Geometry check sheet. Reference: the model listing, model coordinates, mm. Face numbers are marked on the shaded views. A direction names the side the tool comes from. Give positions to 0.01 mm unless a question says otherwise; leave off trailing zeros. Loops run counter-clockwise (first coordinate to the right, second up) from the corner with the lowest first, then second, coordinate; pieces in that order, holes last. Notation, with made-up numbers: (72, 62.5) -> (125, 62.5) arc R7 cw to (125, 70.5) -> close; hole circle Ø4 at (66, 56). An arc over 180 degrees is marked (long way). One line per item, written item: value. Start each with the question number.
(1) Sectioned sample at C-C, the plane x = -34. Record the cut outline in (y, z), then the cut area to 3 significant figures.
(2) Tool access check on the marked faces 3 and 4. Record the directions out of +Z, -Z, +X, -X, +Y, -Y that give a thin tool (end or side, any length) a straight path to the whole face; none if there is none.
(3) Gauge pin test, flat ends, axial feed: pin 1 Ø0.8 at (x, z) = (-15, 0.5) entering from +Y; pin 2 Ø1.1 at (x, z) = (-9.5, 1) entering from +Y; pin 3 Ø10 at (x, y) = (-27, 14) entering from +Z. Record the tip position at first contact, or that the pin passes through.
(4) Scan lines: line 1 along Y through (x, z) = (0, -0.05); line 2 along Y through (x, z) = (0, -1); line 3 along Y through (x, z) = (-4.5, 1.2). Record each from-to range of solid material in increasing order. Write a range as from..to.
(5) Sectioned sample at A-A, the plane y = 0. Record the cut outline in (x, z).
(6) Draft check along Y on the marked faces 1 and 2. Enter one of: pulls with the +Y half, pulls with the -Y half, needs draft (parallel to the pull), parting line crosses it, or undercut.
(7) Sectioned sample at D-D, the plane y = -12.5. Record the cut outline in (x, z).
(8) Sectioned sample at B-B, the plane x = -1.5. Record the cut outline in (y, z).
from build123d import *

# Parameters (mm, degrees)
CYLINDER_R        = 1.1
CYLINDER_DEPTH    = 27
ARRAY018_Y_COUNT  = 2
ARRAY018_Y_PITCH  = 64.8
BOX_W             = 5
BOX_H             = 2.6
BOX_DEPTH         = 10
ARRAY019_X_COUNT  = 3
ARRAY019_X_PITCH  = 11
ARRAY019_Y_COUNT  = 2
ARRAY019_Y_PITCH  = 64.8
ARRAY017_X_COUNT  = 2
ARRAY017_X_PITCH  = 3
ARRAY017_Y_COUNT  = 2
ARRAY017_Y_PITCH  = 64.8
BOX030_W          = 1.8
BOX030_H          = 68
BOX030_DEPTH      = 10
BOX029_W          = 37
BOX029_H          = 1.8
BOX029_DEPTH      = 10
ARRAY016_Y_COUNT  = 2
ARRAY016_Y_PITCH  = 66.2
CYLINDER021_R     = 6
CYLINDER021_DEPTH = 10
CYLINDER022_R     = 7
CYLINDER022_DEPTH = 10
CYLINDER020_R     = 6
CYLINDER020_DEPTH = 10
BOX028_W          = 22
BOX028_H          = 58
BOX028_DEPTH      = 1.5
BOX027_W          = 52
BOX027_H          = 29
BOX027_DEPTH      = 1.5
BOX026_W          = 52
BOX026_H          = 62
BOX026_DEPTH      = 1
FILLET018_R       = 2.5
FILLET019_R       = 10.5
CYLINDER019_W     = 15.5
CYLINDER019_H     = 3.1
CYLINDER019_ANGLE = 90
BOX024_W          = 15.5
BOX024_H          = 37
BOX024_DEPTH      = 3.1
BOX025_W          = 43.5
BOX025_H          = 68
BOX025_DEPTH      = 3.1
FILLET017_R       = 2
CYLINDER018_W     = 15.5
CYLINDER018_H     = 3.1
CYLINDER018_ANGLE = 90
FILLET020_R       = 1


with BuildPart() as array018:
    # Cylinder → Cylinder (new body)
    with BuildSketch(Plane(origin=(-40.5, -32.4, 0.2), x_dir=(0, 0, -1), z_dir=(1, 0, 0))):
        Circle(CYLINDER_R)
    extrude(amount=CYLINDER_DEPTH)

    # Array018 Y: Array018 ×2


with BuildPart() as array018_1:
    add(array018.part)
    with Locations(*[(0, i * ARRAY018_Y_PITCH, 0) for i in range(1, ARRAY018_Y_COUNT)]):
        add(array018.part)


with BuildPart() as array019:
    # Box → Box (new body)
    with BuildSketch(Plane(origin=(-18.5, -33.5, 0.2), x_dir=(1, 0, 0), z_dir=(0, 0, 1))):
        with Locations((2.5, 1.3)):
            Rectangle(BOX_W, BOX_H)
    extrude(amount=BOX_DEPTH)

    # Array019 X: Array019 ×3


with BuildPart() as array019_1:
    add(array019.part)
    with Locations(*[(-i * ARRAY019_X_PITCH, 0, 0) for i in range(1, ARRAY019_X_COUNT)]):
        add(array019.part)

    # Array019 Y: Array019 ×2


with BuildPart() as array019_2:
    add(array019_1.part)
    with Locations(*[(0, i * ARRAY019_Y_PITCH, 0) for i in range(1, ARRAY019_Y_COUNT)]):
        add(array019_1.part)


with BuildPart() as obj1:
    # Sphere001 → Sphere001 (revolve)
    with BuildSketch(Plane(origin=(-10.5, -32.4, 0.2), x_dir=(1, 0, 0), z_dir=(0, -1, 0))):
        with BuildLine():
            ThreePointArc((0, -1.1), (1.1, 0), (0, 1.1))
            Line((0, 1.1), (0, -1.1))
        make_face()
    revolve(axis=Axis((-10.5, -32.4, 0.2), (0, 0, 1)))

    # Array017 X: obj1_2


with BuildPart() as obj1_1:
    add(obj1.part)
    with Locations(*[(-i * ARRAY017_X_PITCH, 0, 0) for i in range(1, ARRAY017_X_COUNT)]):
        add(obj1.part)

    # Array017 Y: obj1_2


with BuildPart() as obj1_2:
    add(obj1_1.part)
    with Locations(*[(0, i * ARRAY017_Y_PITCH, 0) for i in range(1, ARRAY017_Y_COUNT)]):
        add(obj1_1.part)

    # Fusion013: union Array018, Array019
    add(array018_1.part)
    add(array019_2.part)


with BuildPart() as obj2:
    # Box030 → Box030 (new body)
    with BuildSketch(Plane(origin=(-43.5, -34, -1.4), x_dir=(1, 0, 0), z_dir=(0, 0, 1))):
        with Locations((0.9, 34)):
            Rectangle(BOX030_W, BOX030_H)
    extrude(amount=BOX030_DEPTH)


with BuildPart() as obj3:
    # Box029 → Box029 (new body)
    with BuildSketch(Plane(origin=(-43.5, -34, -1.4), x_dir=(1, 0, 0), z_dir=(0, 0, 1))):
        with Locations((18.5, 0.9)):
            Rectangle(BOX029_W, BOX029_H)
    extrude(amount=BOX029_DEPTH)

    # Array016 Y: obj3 ×2


with BuildPart() as obj3_1:
    add(obj3.part)
    with Locations(*[(0, i * ARRAY016_Y_PITCH, 0) for i in range(1, ARRAY016_Y_COUNT)]):
        add(obj3.part)

    # Fusion012: union obj2
    add(obj2.part)


with BuildPart() as obj4:
    # Cylinder021 → Cylinder021 (new body)
    with BuildSketch(Plane(origin=(0, 21.5, -3), x_dir=(1, 0, 0), z_dir=(0, 0, 1))):
        Circle(CYLINDER021_R)
    extrude(amount=CYLINDER021_DEPTH)


with BuildPart() as obj5:
    # Cylinder022 → Cylinder022 (new body)
    with BuildSketch(Plane.XY.offset(-3)):
        Circle(CYLINDER022_R)
    extrude(amount=CYLINDER022_DEPTH)


with BuildPart() as obj6:
    # Cylinder020 → Cylinder020 (new body)
    with BuildSketch(Plane(origin=(0, -21.5, -3), x_dir=(1, 0, 0), z_dir=(0, 0, 1))):
        Circle(CYLINDER020_R)
    extrude(amount=CYLINDER020_DEPTH)

    # Fusion009: union obj4, obj5
    add(obj4.part)
    add(obj5.part)


with BuildPart() as partcut2:
    # Box028 → Box028 (new body)
    with BuildSketch(Plane(origin=(-39, -29, -0.8), x_dir=(1, 0, 0), z_dir=(0, 0, 1))):
        with Locations((11, 29)):
            Rectangle(BOX028_W, BOX028_H)
    extrude(amount=BOX028_DEPTH)


with BuildPart() as partcuts:
    # Box027 → Box027 (new body)
    with BuildSketch(Plane(origin=(-41, -14.5, -0.8), x_dir=(1, 0, 0), z_dir=(0, 0, 1))):
        with Locations((26, 14.5)):
            Rectangle(BOX027_W, BOX027_H)
    extrude(amount=BOX027_DEPTH)

    # Fusion008: union PartCut2
    add(partcut2.part)


with BuildPart() as fillet019:
    # Box026 → Box026 (new body)
    with BuildSketch(Plane(origin=(-41, -31, 0.7), x_dir=(1, 0, 0), z_dir=(0, 0, 1))):
        with Locations((26, 31)):
            Rectangle(BOX026_W, BOX026_H)
    extrude(amount=BOX026_DEPTH)

    # Fillet018
    fillet018_edges = [fillet019.edges().sort_by_distance(p)[0] for p in [
        (-41, -31, 1.2),
        (-41, 31, 1.2),
    ]]
    fillet(fillet018_edges, radius=FILLET018_R)

    # Fillet019
    fillet019_edges = [fillet019.edges().sort_by_distance(p)[0] for p in [
        (11, -31, 1.2),
        (11, 31, 1.2),
    ]]
    fillet(fillet019_edges, radius=FILLET019_R)


with BuildPart() as obj7:
    # Cylinder019 → Cylinder019 (revolve)
    with BuildSketch(Plane(origin=(0, -18.5, -1.4), x_dir=(0, -1, 0), z_dir=(-1, 0, 0))):
        with Locations((7.75, 1.55)):
            Rectangle(CYLINDER019_W, CYLINDER019_H)
    revolve(axis=Axis((0, -18.5, -1.4), (0, 0, 1)), revolution_arc=CYLINDER019_ANGLE)


with BuildPart() as obj8:
    # Box024 → Box024 (new body)
    with BuildSketch(Plane(origin=(0, -18.5, -1.4), x_dir=(1, 0, 0), z_dir=(0, 0, 1))):
        with Locations((7.75, 18.5)):
            Rectangle(BOX024_W, BOX024_H)
    extrude(amount=BOX024_DEPTH)


with BuildPart() as fillet017:
    # Box025 → Box025 (new body)
    with BuildSketch(Plane(origin=(-43.5, -34, -1.4), x_dir=(1, 0, 0), z_dir=(0, 0, 1))):
        with Locations((21.75, 34)):
            Rectangle(BOX025_W, BOX025_H)
    extrude(amount=BOX025_DEPTH)

    # Fillet017
    fillet017_edges = [fillet017.edges().sort_by_distance(p)[0] for p in [
        (-43.5, -34, 0.15),
        (-43.5, 34, 0.15),
    ]]
    fillet(fillet017_edges, radius=FILLET017_R)


with BuildPart() as obj9:
    # Cylinder018 → Cylinder018 (revolve)
    with BuildSketch(Plane(origin=(0, 18.5, -1.4), x_dir=(1, 0, 0), z_dir=(0, -1, 0))):
        with Locations((7.75, 1.55)):
            Rectangle(CYLINDER018_W, CYLINDER018_H)
    revolve(axis=Axis((0, 18.5, -1.4), (0, 0, 1)), revolution_arc=CYLINDER018_ANGLE)

    # Fusion007: union obj7, obj8, Fillet017
    add(obj7.part)
    add(obj8.part)
    add(fillet017.part)

    # Cut030: cut Fillet019
    add(fillet019.part, mode=Mode.SUBTRACT)

    # Cut031: cut PartCuts
    add(partcuts.part, mode=Mode.SUBTRACT)

    # Cut032: cut obj6
    add(obj6.part, mode=Mode.SUBTRACT)

    # Cut033: cut obj3
    add(obj3_1.part, mode=Mode.SUBTRACT)

    # Fillet020
    fillet020_edges = [obj9.edges().sort_by_distance(p)[0] for p in [
        (-6.5, 34, 0.15),
        (-6.5, -34, 0.15),
        (-41.7, -32.2, 0.15),
        (-41.7, 32.2, 0.15),
    ]]
    fillet(fillet020_edges, radius=FILLET020_R)

    # Cut: cut obj1
    add(obj1_2.part, mode=Mode.SUBTRACT)


solid = obj9.part
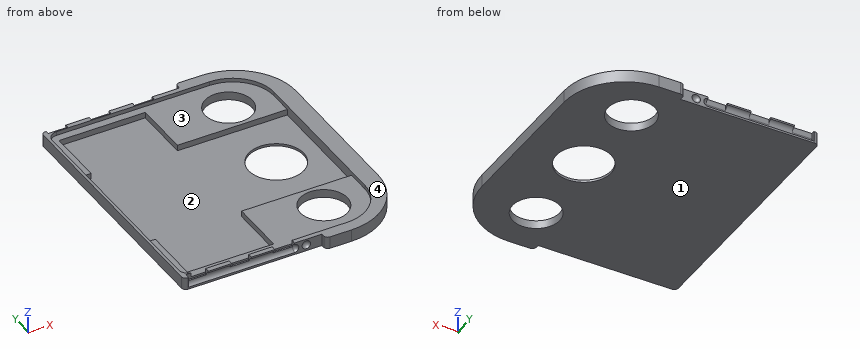
Calculated:
1. outline: (-32.2, -1.4) -> (32.2, -1.4) -> (32.2, -0.88) arc R1.1 cw to (32.2, 1.28) -> (32.2, 1.7) -> (31, 1.7) -> (31, 0.7) -> (29, 0.7) -> (29, -0.8) -> (-29, -0.8) -> (-29, 0.7) -> (-31, 0.7) -> (-31, 1.7) -> (-32.2, 1.7) -> (-32.2, 1.28) arc R1.1 cw to (-32.2, -0.88) -> close
1. area: 47.7 mm2
2. face 3: +Z
2. face 4: +Z, +X, -X, +Y, -Y
3. pin 1: stops at y = 31.3
3. pin 2: stops at y = 32.2
3. pin 3: stops at z = -0.8
4. line 1: y = -34..-27.5, -15.5..-14.5, 14.5..15.5, 27.5..34
4. line 2: y = -34..-27.5, -15.5..-7, 7..15.5, 27.5..34
4. line 3: y = -34..-31, 31..34
5. outline: (-41.7, -1.4) -> (-7, -1.4) -> (-7, -0.8) -> (-41, -0.8) -> (-41, 1.7) -> (-41.7, 1.7) -> close; (7, -1.4) -> (15.5, -1.4) -> (15.5, 1.7) -> (11, 1.7) -> (11, -0.8) -> (7, -0.8) -> close
6. face 1: needs draft
6. face 2: undercut
7. outline: (-41.7, -1.4) -> (15.5, -1.4) -> (15.5, 1.7) -> (11, 1.7) -> (11, -0.8) -> (-41, -0.8) -> (-41, 1.7) -> (-41.7, 1.7) -> close
8. outline: (-34, -1.4) -> (-27.31, -1.4) -> (-27.31, 0.7) -> (-31, 0.7) -> (-31, 1.7) -> (-34, 1.7) -> close; (-15.69, -1.4) -> (-6.84, -1.4) -> (-6.84, -0.8) -> (-14.5, -0.8) -> (-14.5, 0.7) -> (-15.69, 0.7) -> close; (6.84, -1.4) -> (15.69, -1.4) -> (15.69, 0.7) -> (14.5, 0.7) -> (14.5, -0.8) -> (6.84, -0.8) -> close; (27.31, -1.4) -> (34, -1.4) -> (34, 1.7) -> (31, 1.7) -> (31, 0.7) -> (27.31, 0.7) -> close
